Could you check a few things on this model? Use its own coordinates, in mm. A direction names the side the tool comes from. Round coordinates to 2 decimals unless told otherwise and drop trailing zeros. Loops run counter-clockwise (first coordinate to the right, second up) from the corner with the lowest first, then second, coordinate; pieces in that order, holes last. Notation, with made-up numbers: (5.5, -0.5) -> (64.5, -0.5) arc R22 cw to (64.5, 19.5) -> close; hole circle Ø2 at (0, 46). An arc over 180 degrees is marked (long way). Write each question's results on one line, items separated by ' | '.
from build123d import *

# Parameters (mm, degrees)
F0_R          = 14.48
F1_DEPTH      = 25
F2_R          = 12.5
F3_DEPTH      = 22
F4_R          = 9
F5_DEPTH      = 3
F6_R          = 12.5
F7_DEPTH      = 1
F8_R          = 12.95
F9_DEPTH      = 10
F10_R         = 10.8
F11_DEPTH     = 11
F12_S5_R      = 10.8
F12_T6_DEPTH  = 19
F12_S11_R     = 9
F12_T12_DEPTH = 19


# Not quite as in the source:
# - a fillet or chamfer that OpenCascade refuses, or shapes differently, is made with other operations: its cross-section is extruded or revolved along the edge and cut away or added


with BuildPart() as f1:
    # F0 (on Top) → F1 (new body)
    with BuildSketch(Plane.XY):
        Circle(F0_R)
    extrude(amount=F1_DEPTH)

    # F2 (on face) → F3 (cut)
    with BuildSketch(Plane.XY.offset(25)):
        Circle(F2_R)
    extrude(amount=-F3_DEPTH, mode=Mode.SUBTRACT)

    # F4 (on face) → F5 (cut, through all)
    with BuildSketch(Plane(origin=(0, 0, 0), x_dir=(1, 0, 0), z_dir=(0, 0, -1))):
        Circle(F4_R)
    extrude(amount=-F5_DEPTH, mode=Mode.SUBTRACT)

    # F6 (on face) → F7 (join)
    with BuildSketch(Plane.XY.offset(25)):
        Circle(F6_R)
    extrude(amount=-F7_DEPTH)

    # F8 (on face) → F9 (join)
    with BuildSketch(Plane.XY.offset(25)):
        Circle(F8_R)
    extrude(amount=F9_DEPTH)

    # F10 (on face) → F11 (cut, through all)
    with BuildSketch(Plane.XY.offset(35)):
        Circle(F10_R)
    extrude(amount=-F11_DEPTH, mode=Mode.SUBTRACT)

    # F12: chamfer of 5 on 3 edges, made by hand


with BuildPart() as f12_tool2:
    # F12_s3 → F12_t4 (revolve)
    with BuildSketch(Plane.XZ):
        Polygon((12.5, 19), (7.5, 24), (12.5, 24), align=None)
    revolve(axis=Axis((0, 0, 24), (0, 0, 1)))

    # F12_s5 → F12_t6 (cut, symmetric)
    with BuildSketch(Plane.XY.offset(21.5)):
        Circle(F12_S5_R)
    extrude(amount=F12_T6_DEPTH, both=True, mode=Mode.SUBTRACT)


with BuildPart() as f1_1:
    add(f1.part)

    # F12_t1: union F12_tool2
    add(f12_tool2.part)


with BuildPart() as f12_tool8:
    # F12_s9 → F12_t10 (revolve)
    with BuildSketch(Plane.XZ):
        Polygon((7.5, 3), (12.5, 8), (12.5, 3), align=None)
    revolve(axis=Axis((0, 0, 3), (0, 0, 1)))

    # F12_s11 → F12_t12 (cut, symmetric)
    with BuildSketch(Plane.XY.offset(5.5)):
        Circle(F12_S11_R)
    extrude(amount=F12_T12_DEPTH, both=True, mode=Mode.SUBTRACT)


with BuildPart() as f1_2:
    add(f1_1.part)

    # F12_t7: union F12_tool8
    add(f12_tool8.part)


solid = f1_2.part
1) I need wall thicknesses on line 1 (Y direction, x = 0, z = 2.15); line 2 (Y direction, x = 0, z = 12); line 3 (X direction, y = 6.5, z = 8). Which ranges of each line are inside material? Lowest first, please.
Model answer:
line 1: y = -14.48 to -9, 9 to 14.48 | line 2: y = -14.48 to -12.5, 12.5 to 14.48 | line 3: x = -12.94 to -10.68, 10.68 to 12.94
2) I want a section at A-A, the plane x = 0. Write out the boundary of the cut face in (y, z).
Model answer:
outline: (-14.48, 0) -> (-9, 0) -> (-9, 4.5) -> (-12.5, 8) -> (-12.5, 19) -> (-10.8, 20.7) -> (-10.8, 35) -> (-12.95, 35) -> (-12.95, 25) -> (-14.48, 25) -> close; (9, 0) -> (14.48, 0) -> (14.48, 25) -> (12.95, 25) -> (12.95, 35) -> (10.8, 35) -> (10.8, 20.7) -> (12.5, 19) -> (12.5, 8) -> (9, 4.5) -> close
3) If we mould it in two halves opening along Y, with no side actions, what happens to faces 4 (the flat face through (-7, -6, 0)), 5 (the cylindrical face through (-3.139, -14.136, 12.325)), 6 (the conical face through (8.793, 2.769, 4.719))? For each: released by +Y, released by -Y, zero draft, split by the parting line, or undercut.
Model answer:
face 4: zero draft | face 5: split by the parting line | face 6: undercut
4) I want a section at D-D, the plane z = 10. Write out the boundary of the cut face in (x, y).
Model answer:
outline: circle Ø28.96 at (0, 0); hole circle Ø25 at (0, 0)
5) I'm going to push flat-ended pins straight in: pin 1 (1 mm diameter, centred on y = 2.5, z = 13.5, fed in from +X); pin 2 (10 mm diameter, centred on x = -10, z = 30.5, fed in from -Y); pin 3 (1.5 mm diameter, centred on x = 11.5, z = 13.5, fed in from -Y); pin 4 (11 mm diameter, centred on x = 0, y = 0, fed in from -Z). Where does each tip first touch, or does it pass through?
Model answer:
pin 1: stops at x = 14.34 | pin 2: stops at y = -11.95 | pin 3: stops at y = -9.7 | pin 4: passes through
6) For faces 1 (the cylindrical face through (11.923, 3.755, 13.577)), 2 (the cylindrical face through (8.584, 2.703, 2.282)), 3 (the cylindrical face through (-2.81, -12.64, 29.93)), which set-ups out of +Z, -Z, +X, -X, +Y, -Y let a thin tool reach every point of the face, with its end or its side?
Model answer:
face 1: none | face 2: +Z, -Z | face 3: +Z
7) I want a section at C-C, the plane z = 27. Write out the boundary of the cut face in (x, y), plus the area to 3 significant figures.
Model answer:
outline: circle Ø25.9 at (0, 0); hole circle Ø21.6 at (0, 0) | area: 160 mm2
